Could you check a few things on this model? Use its own coordinates, in mm. A direction names the side the tool comes from. Round coordinates to 2 decimals unless told otherwise and drop trailing zeros. Loops run counter-clockwise (first coordinate to the right, second up) from the corner with the lowest first, then second, coordinate; pieces in that order, holes last.
from build123d import *

# Parameters (mm, degrees)
SKETCH8_W           = 75
SKETCH8_H           = 9
BOSS_EXTRUDE5_DEPTH = 52
BOSS_EXTRUDE6_DEPTH = 8


with BuildPart() as part:
    # Sketch8 → Boss-Extrude5 (new body)
    with BuildSketch(Plane(origin=(0, 0, 0), x_dir=(1, 0, 0), z_dir=(0, 1, 0))):
        with BuildLine():
            Line((-4.5, 21.5), (-4.5, 4.5))
            Line((-4.5, 4.5), (4.5, 4.5))
            Line((4.5, 4.5), (4.5, 21.5))
            Line((4.5, 21.5), (4.5, 21.944512863))
            ThreePointArc((4.5, 21.944512863), (17.783419244, 29.914047854), (23, 44.5))
            Line((23, 44.5), (15, 44.5))
            ThreePointArc((15, 44.5), (0, 29.5), (-15, 44.5))
            Line((-15, 44.5), (-23, 44.5))
            ThreePointArc((-23, 44.5), (-17.783419244, 29.914047854), (-4.5, 21.944512863))
            Line((-4.5, 21.944512863), (-4.5, 21.5))
        make_face()
        Rectangle(SKETCH8_W, SKETCH8_H)
    extrude(amount=-BOSS_EXTRUDE5_DEPTH)

    # Sketch9 → Boss-Extrude6 (add)
    with BuildSketch(Plane(origin=(0, -30, 0), x_dir=(-1, 0, 0), z_dir=(0, -1, 0))):
        with BuildLine():
            Line((23, 44.5), (37.5, 4.5))
            Line((37.5, 4.5), (4.5, 4.5))
            Line((4.5, 4.5), (4.5, 21.944512863))
            ThreePointArc((4.5, 21.944512863), (17.783419244, 29.914047854), (23, 44.5))
        make_face()
    extrude(amount=-BOSS_EXTRUDE6_DEPTH)


solid = part.part
Item 1: We'd pull the mould along Z, two halves only. Please class faces 5 (the cylindrical face through (-17.923, -40.846, -30.086)), 6 (the flat face through (-37.5, -26, 0)), 7 (the cylindrical face through (0.33, -25.636, -29.504)): released by +Z, released by -Z, zero draft, split by the parting line, or undercut.
Results list:
face 5: undercut
face 6: zero draft
face 7: released by -Z
Item 2: If we section it at C-C, the plane z = -33.5: Please give me the cut outline in (x, y).
Results list:
outline: (-26.99, -30) - (-20.2, -30) - (-20.2, -52) - (-10.2, -52) - (-10.2, 0) - (-20.2, 0) - (-20.2, -22) - (-26.99, -22) - close; (10.2, -52) - (20.2, -52) - (20.2, 0) - (10.2, 0) - close
Item 3: Will these pins go through, and if not, where does the flat tip stop? pin 1 (3 mm diameter, centred on x = -11, z = -21, fed in from -Y); pin 2 (4 mm diameter, centred on y = -18.5, z = -23, fed in from -X); pin 3 (8.5 mm diameter, centred on y = -11.5, z = -15, fed in from -X).
Results list:
pin 1: stops at y = -30
pin 2: stops at x = -12.2
pin 3: stops at x = -4.5
Item 4: If I drill on line 1 along X through (y, z) = (-47.5, -21); line 2 along Z through (x, y) = (12, -34); line 3 along Y through (x, z) = (-22.5, -36.5), over which ranges is the centre line in solid material (lowest first)?
Results list:
line 1: x = -4.5 to 4.5
line 2: z = -35.5 to -24.88, -4.5 to 4.5
line 3: y = -30 to -22
Item 5: If we section it at D-D, the plane x = -31: Please give me the cut outline in (y, z).
Results list:
outline: (-52, -4.5) - (-30, -4.5) - (-30, -22.43) - (-22, -22.43) - (-22, -4.5) - (0, -4.5) - (0, 4.5) - (-52, 4.5) - close
Item 6: If we section it at A-A, the plane x = 12.5: Please give me the cut outline in (y, z), then the cut area to 3 significant figures.
Results list:
outline: (-52, -36.21) - (0, -36.21) - (0, -25.19) - (-52, -25.19) - close; (-52, -4.5) - (0, -4.5) - (0, 4.5) - (-52, 4.5) - close
area: 1,040 mm2
Item 7: For faces 1 (the flat face through (-4.5, -11, -13)), 2 (the flat face through (4.5, -26, -13)), 3 (the flat face through (19, -26, -44.5)), 4 (the flat face through (-21, -41, -4.5)), which set-ups out of +Z, -Z, +X, -X, +Y, -Y let a thin tool reach every point of the face, with its end or its side?
Results list:
face 1: -X, +Y
face 2: +X, +Y, -Y
face 3: -Z, +X, -X, +Y, -Y
face 4: -X, -Y
Item 8: If we section it at B-B, the plane y = -39.5: Please give me the cut outline in (x, z), then the cut area to 3 significant figures.
Results list:
outline: (-37.5, -4.5) - (-4.5, -4.5) - (-4.5, -21.94) arc R23 ccw to (-23, -44.5) - (-15, -44.5) arc R15 cw to (15, -44.5) - (23, -44.5) arc R23 ccw to (4.5, -21.94) - (4.5, -4.5) - (37.5, -4.5) - (37.5, 4.5) - (-37.5, 4.5) - close
area: 1,310 mm2
